from build123d import *
from build123d.topology import SkipClean

# Parameters (mm, degrees)
CROQUIS1_R                 = 17.1
CROQUIS1_R_2               = 14.1
SALIENTE_EXTRUIR1_DEPTH    = 4.5
CORTAR_EXTRUIR1_REACH      = 27.803
CROQUIS2_W                 = 15.420651877
CROQUIS2_H                 = 7.2
CROQUIS54_W                = 3
CROQUIS54_H                = 19
REVOLUCI_N1_ANGLE          = 150
CORTAR_BARRER2_PROFILE_R   = 2.25
CHAFL_N3_SIZE              = 5
CORTAR_EXTRUIR2_REACH      = 27.982
CORTAR_EXTRUIR2_END_RADIUS = 16.1
CROQUIS61_R                = 3
CORTAR_EXTRUIR3_DEPTH      = 26.982109266
CORTAR_EXTRUIR3_DEPTH_BACK = 26.982109266
CORTAR_EXTRUIR4_REACH      = 41.067
CORTAR_EXTRUIR4_END_RADIUS = 14.1
CROQUIS63_R                = 0.75
CROQUIS64_R                = 1.25
CORTAR_EXTRUIR5_DEPTH      = 0.5
CORTAR_EXTRUIR6_START      = -11
CROQUIS65_W                = 2.8
CROQUIS65_H                = 19.872981168
CORTAR_EXTRUIR6_DEPTH      = 11


with BuildPart() as part:
    # Croquis1 → Saliente-Extruir1 (new, symmetric)
    with BuildSketch(Plane(origin=(0, 0, 0), x_dir=(1, 0, 0), z_dir=(0, 1, 0))):
        with Locations(Location((0, 0, 0), (0, 0, 270))):
            Circle(CROQUIS1_R)
        with Locations(Location((0, 0, 0), (0, 0, 270))):
            Circle(CROQUIS1_R_2, mode=Mode.SUBTRACT)
    extrude(amount=SALIENTE_EXTRUIR1_DEPTH, both=True)

    # Croquis2 → Cortar-Extruir1 (cut, up to next)
    with BuildSketch(Plane(origin=(0, 4.5, 0), x_dir=(1, 0, 0), z_dir=(0, 1, 0)), mode=Mode.PRIVATE) as cortar_extruir1_sk1:
        with Locations((15.870282115, 0)):
            Rectangle(CROQUIS2_W, CROQUIS2_H)
    cortar_extruir1_tool1 = extrude(cortar_extruir1_sk1.sketch, amount=-CORTAR_EXTRUIR1_REACH, mode=Mode.PRIVATE) & part.part
    add(cortar_extruir1_tool1.solids().sort_by_distance((15.870282, 4.5, 0))[0], mode=Mode.SUBTRACT)

    # Croquis54 → Revolución1 (revolve, symmetric)
    with SkipClean():  # the faces are left unmerged after this step: merging them gives an invalid solid
        with BuildSketch(Plane.XY) as revoluci_n1_sk:
            with Locations((-15.6, 0)):
                Rectangle(CROQUIS54_W, CROQUIS54_H)
        revolve(axis=Axis((0, -13.582020258, 0), (0, 1, 0)), revolution_arc=REVOLUCI_N1_ANGLE / 2)
        revolve(revoluci_n1_sk.sketch, axis=Axis((0, -13.582020258, 0), (0, -1, 0)), revolution_arc=REVOLUCI_N1_ANGLE / 2)
    add(part.part.scale(1), mode=Mode.REPLACE)  # the faces are merged on a copy

    # Cortar-Barrer2: sweep along a path in Croquis12
    with BuildLine(Plane(origin=(0, 0, 0), x_dir=(1, 0, 0), z_dir=(0, 1, 0))) as cortar_barrer2_path:
        CenterArc((0, 0), 14.1, 0, 360)
    # Cortar-Barrer2 profile (on start of the path) → Cortar-Barrer2 (sweep, cut)
    with BuildSketch(Plane(origin=(14.1, 0, 0), x_dir=(-1, 0, 0), z_dir=(0, 0, -1))):
        Circle(CORTAR_BARRER2_PROFILE_R)
    sweep(path=cortar_barrer2_path.line, mode=Mode.SUBTRACT)

    # Chaflán3
    chafl_n3_edges = [part.edges().sort_by_distance(p)[0] for p in [
        (-4.037577104, -9.5, -15.06844289),
        (-4.037577104, 9.5, -15.06844289),
        (-4.037577104, -9.5, 15.06844289),
        (-4.037577104, 9.5, 15.06844289),
    ]]
    chamfer(chafl_n3_edges, length=CHAFL_N3_SIZE - 0.0001)  # a hair under: the kernel refuses the full size

    # Cortar-Extruir2: up to this cylinder (the profile starts inside it)
    cortar_extruir2_end = Plane(origin=(0, 0, 0), z_dir=(0, -1, 0)) * Cylinder(CORTAR_EXTRUIR2_END_RADIUS, 89.164, mode=Mode.PRIVATE)
    # Croquis61 → Cortar-Extruir2 (cut, up to the surface)
    with BuildSketch(Plane(origin=(0, 0, 0), x_dir=(0, 0, -1), z_dir=(1, 0, 0)), mode=Mode.PRIVATE) as cortar_extruir2_sk1:
        Circle(CROQUIS61_R)
    cortar_extruir2_tool1 = extrude(cortar_extruir2_sk1.sketch, amount=-CORTAR_EXTRUIR2_REACH, mode=Mode.PRIVATE) & cortar_extruir2_end
    add(cortar_extruir2_tool1.solids().sort_by_distance((0, 0, 0))[0], mode=Mode.SUBTRACT)

    # Croquis62 → Cortar-Extruir3 (cut, two sides: drawn at the far end of the back side and taken through both)
    with BuildSketch(Plane(origin=(0, 0, 0), x_dir=(0, 0, -1), z_dir=(1, 0, 0)).offset(-CORTAR_EXTRUIR3_DEPTH_BACK)):
        Polygon((-3.6, 1.5), (-3.6, 0), (3.6, 0), (3.6, 1.5), (19.353781031, 1.5), (19.353781031, 12.340609049), (-20.692074401, 12.340609049), (-20.692074401, 1.5), align=None)
    extrude(amount=CORTAR_EXTRUIR3_DEPTH + CORTAR_EXTRUIR3_DEPTH_BACK, mode=Mode.SUBTRACT)

    # Cortar-Extruir4: up to this cylinder (the profile starts outside it)
    with SkipClean():  # the faces are left unmerged after this step: merging them gives an invalid solid
        cortar_extruir4_end = Plane(origin=(0, -5, 0), z_dir=(0, -1, 0)) * Cylinder(CORTAR_EXTRUIR4_END_RADIUS, 111.334, mode=Mode.PRIVATE)
        # Croquis63 → Cortar-Extruir4 (cut, up to the surface)
        with BuildSketch(Plane(origin=(-17.1, 0, 0), x_dir=(0, -1, 0), z_dir=(-1, 0, 0)), mode=Mode.PRIVATE) as cortar_extruir4_sk1:
            with Locations(Location((5, 0, 0), (0, 0, 90))):
                Circle(CROQUIS63_R)
        cortar_extruir4_tool1 = extrude(cortar_extruir4_sk1.sketch, amount=-CORTAR_EXTRUIR4_REACH, mode=Mode.PRIVATE) - cortar_extruir4_end
        add(cortar_extruir4_tool1.solids().sort_by_distance((-17.1, -5, 0))[0], mode=Mode.SUBTRACT)

    # Croquis64 → Cortar-Extruir5 (cut)
    with SkipClean():  # the faces are left unmerged after this step: merging them gives an invalid solid
        with BuildSketch(Plane(origin=(-17.1, 0, 0), x_dir=(0, -1, 0), z_dir=(-1, 0, 0))):
            with Locations(Location((5, 0, 0), (0, 0, 90))):
                Circle(CROQUIS64_R)
        extrude(amount=-CORTAR_EXTRUIR5_DEPTH, mode=Mode.SUBTRACT)

    # Croquis65 → Cortar-Extruir6 (cut)
    with SkipClean():  # the faces are left unmerged after this step: merging them gives an invalid solid
        with BuildSketch(Plane(origin=(0, 1.5, 0), x_dir=(1, 0, 0), z_dir=(0, 1, 0)).offset(CORTAR_EXTRUIR6_START)):
            with Locations((15.316758059, 0)):
                Rectangle(CROQUIS65_W, CROQUIS65_H)
        extrude(amount=CORTAR_EXTRUIR6_DEPTH, mode=Mode.SUBTRACT)


solid = part.part
Read the model definition and answer for the solid it produces. Units are mm, in the model's axes. A direction names the side the tool comes from. Give positions to 0.01 mm unless a question says otherwise; leave off trailing zeros. Loops run counter-clockwise (first coordinate to the right, second up) from the corner with the lowest first, then second, coordinate; pieces in that order, holes last. Notation, with made-up numbers: (81, 88) - (110, 88) arc R16 cw to (110, 93) - close; hole circle Ø9 at (84.25, 35). An arc over 180 degrees is marked (long way). Answer as CSV lines item,"result". Start each with the question number.
1) Each of these flat-tipped pins is pushed along its axis until it touches: pin 1 Ø2 at (x, y) = (-5, -2) entering from +Z; pin 2 Ø1.5 at (y, z) = (-5, 12) entering from -X; pin 3 Ø4 at (x, z) = (5.5, 13.5) entering from -Y. Where does it stop, or does it pass through?
2) Find section C-C (y = -7). Write down the section's boundary in (x, z), then the cut area to 3 significant figures.
3) Straight lines are drawn through the part: L1, parallel to Y at x = -15.45, z = 0; L2, parallel to Y at x = -16.85, z = 0; L3, parallel to X at y = -4.25, z = -11. For each, find the intervals that lie inside material, in ascending order. Write a range as from..to.
4) Which of the six approach directions +Z, -Z, +X, -X, +Y, -Y give full straight-line access (tool end or side, diameter ignored) to faces 1 (the face through (-6.375, -7.035, 13.996)), 2 (the face through (-16.854, -5.479, 1.155)), 3 (the face through (-16, 1, -3.6)), 4 (the face through (-16.1, -1.8, 0))?
5) Find section B-B (y = -0.5). Write down the section's boundary in (x, z).
6) Find section A-A (y = -5). Write down the section's boundary in (x, z).
Findings below:
1,pin 1,"z = 16.63"
1,pin 2,"x = -12.88"
1,pin 3,"y = -4.5"
2,outline,"(-6.79, -15.69) - (-6.01, -12.76) arc R14.1 cw to (-6.01, 12.76) - (-6.79, 15.69) arc R17.1 ccw to start"
2,area,"107 mm^2"
3,L1,"-9.5..-5.75, -4.25..-3"
3,L2,"-9.5..-6.25, -3.75..0"
3,L3,"-13.09..-8.82, 8.82..13.09"
4,face 1,"+Z, +X, -Y"
4,face 2,"-X"
4,face 3,"+X, -X, +Y"
4,face 4,"+X, +Y"
5,outline,"(13.92, -9.94) - (13.92, -8.47) arc R16.29 cw (long way) to (13.92, 8.47) - (13.92, 9.94) arc R17.1 ccw (long way) to start"
6,outline,"(-17.05, -1.25) arc R17.1 ccw to (-4.91, -16.38) - (-4.13, -13.48) arc R14.1 cw to (-14.08, -0.75) - (-16.6, -0.75) - (-16.6, -1.25) - close; (-17.05, 1.25) - (-16.6, 1.25) - (-16.6, 0.75) - (-14.08, 0.75) arc R14.1 cw to (-4.13, 13.48) - (-4.91, 16.38) arc R17.1 ccw to start"
